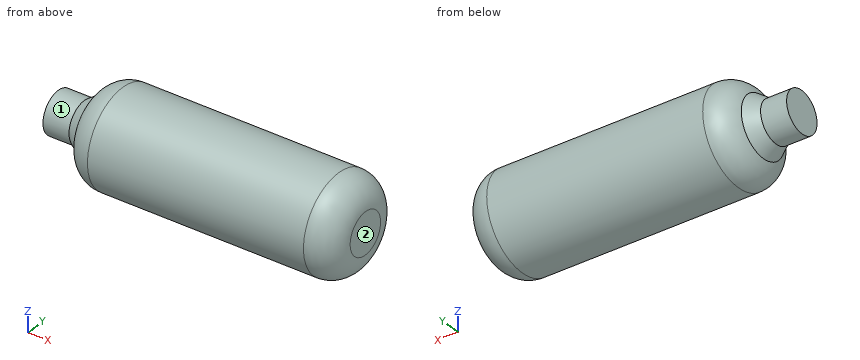
from build123d import *

# Parameters (mm, degrees)
F0_R     = 9
F1_DEPTH = 50.8
F2_R     = 5.08
F3_DEPTH = 7


# Not quite as in the source:
# - a fillet or chamfer that OpenCascade refuses, or shapes differently, is made with other operations: its cross-section is extruded or revolved along the edge and cut away or added


with BuildPart() as f1:
    # F0 (on Right) → F1 (new body)
    with BuildSketch(Plane.YZ):
        Circle(F0_R)
    extrude(amount=F1_DEPTH)

    # F2
    f2_edges = [f1.edges().sort_by_distance(p)[0] for p in [
        (50.8, -9, 0),
        (0, -9, 0),
    ]]
    fillet(f2_edges, radius=F2_R)

    # F3 (add): a face of the model
    f3_faces = [f1.faces().sort_by_distance(p)[0] for p in [
        (0, 0, 0),
    ]]
    extrude(f3_faces, amount=F3_DEPTH)

    # F4: chamfer of 2.54 on 1 edges, made by hand

    # F4_s1 → F4_t2 (revolve)
    with BuildSketch(Plane.XY):
        with BuildLine():
            Line((0.2905300688, 5.6133333333), (-2.1042048969, 3.92))
            Line((-2.1042048969, 3.92), (0, 3.92))
            ThreePointArc((0, 3.92), (0.0794974837, 4.8151952776), (0.2905300688, 5.6133333333))
        make_face()
    revolve(axis=Axis((0, 0, 0), (1, 0, 0)))


solid = f1.part
Design review of the part built by this model. Coordinates are the model's own, in mm. Face numbers are marked on the shaded views. A direction names the side the tool comes from. Coordinates: 2 decimals unless noted, no trailing zeros. Loops run counter-clockwise (first coordinate to the right, second up) from the corner with the lowest first, then second, coordinate; pieces in that order, holes last. Notation, with made-up numbers: (20, 15) -> (52, 15) arc R10 cw to (52, 20) -> close; hole circle Ø3 at (21.25, 67.25). An arc over 180 degrees is marked (long way). Use a Markdown table: item, result. Add a question column.
Item 1: Machinability: for the marked faces 1 and 2, which of the approach directions +Z, -Z, +X, -X, +Y, -Y give a long, thin tool a straight path to every point of the face, cutting with its end or side? Answer none if there is none.
Item 2: Wall thickness on L1, parallel to Y at x = 8.5, z = -3.5; L2, parallel to Y at x = 24.5, z = -7.5; L3, parallel to Z at x = 30, y = -4.25: over which ranges is each line inside the solid? List them lowest first. Write a range as from..to.
Item 3: We need section A-A, the plane x = 23. Write out the cut boundary in (y, z).
Item 4: Clearance check with flat-ended pins moving along their axes: P1, Ø8, axis at y = 6, z = -1, coming from the +X side; P2, Ø2, axis at x = 19.5, y = 1.5, coming from the -Z side; P3, Ø2, axis at x = 22, z = 7, coming from the +Y side; P4, Ø10, axis at x = 10, z = -6.5, coming from the +Y side. State where each tip first meets the part, or that it passes through.
Numbers:
| question | item | result |
|---|---|---|
| 1 | face 1 | -X |
| 1 | face 2 | +Z, -Z, +X, +Y, -Y |
| 2 | L1 | y = -8.29..8.29 |
| 2 | L2 | y = -4.97..4.97 |
| 2 | L3 | z = -7.93..7.93 |
| 3 | outline | circle Ø18 at (0, 0) |
| 4 | P1 | stops at x = 50.8 |
| 4 | P2 | stops at z = -8.99 |
| 4 | P3 | stops at y = 6.71 |
| 4 | P4 | stops at y = 8.87 |
